Read the model definition and answer for the solid it produces. Units are mm, in the model's axes. A direction names the side the tool comes from. Give positions to 0.01 mm unless a question says otherwise; leave off trailing zeros. Order: outer loops, then holes, each group sorted by start corner. A loop starts at its lowest first (then second) coordinate and runs counter-clockwise, first axis right, second up. Notation, with made-up numbers: (62.5, 18.5) - (104.5, 18.5) arc R12 ccw to (104.5, 36.5) - close; hole circle Ø4 at (-12.5, 78). An arc over 180 degrees is marked (long way). Write each question's results on one line, items separated by ' | '. Start each with the question number.
Q1. A tool of negligible diameter and unlimited length cuts with its end or side. For faces 4 (the face through (0, 18.3, 0)), 5 (the face through (0.596, 5.315, -1.337)), 6 (the face through (-12, 1, 1.067)), from which of +Z, -Z, +X, -X, +Y, -Y can it reach the whole face along a straight path? Write none if from no direction.
Q2. Find the intervals of material crossed by line 1 along Y through (x, z) = (0, 1.45); line 2 along Y through (x, z) = (0, 0.25); line 3 along X through (y, z) = (1.75, 0.15), in increasing order. Write a range as from..to.
Q3. For a pull along Y with two mould halves and no side action, classify faces 1 (the face through (2.859, -2.797, -0.022)), 2 (the face through (-3, 6, -1.6)), 3 (the face through (-0.8, 15, 0)) as +Y half, -Y half, draft (parallel to the pull), parting line (faces both ways), or undercut.
Q4. Find section D-D on z = -0.1. Count the separate pieces of the cut face and the enclosed holes in it, and give its area (3 significant figures).
Q5. Find section A-A on x = -8. Give the vertices of the cut face in (y, z), and give its area (3 significant figures).
Q6. Flat-ended cylindrical pins translate along their axes: P1, Ø1.1, axis at y = -1.5, z = -0.5, coming from the -X side; P2, Ø0.7, axis at y = 17.5, z = -0.5, coming from the +X side; P3, Ø1.1, axis at y = -2, z = 0.5, coming from the +X side. Find the tip coordinate at first contact, or state that the pin passes through.
Q7. Find section C-C on x = -14.5. Give the vertices of the cut face in (y, z), and give its area (3 significant figures).
Autodesk Inventor part; units mm, degrees
ref_plane "YZ Plane" through (0, 0, 0) normal (1, 0, 0) x (0, 1, 0)
ref_plane "XZ Plane" through (0, 0, 0) normal (0, 1, 0) x (-1, 0, 0)
ref_plane "XY Plane" through (0, 0, 0) normal (0, 0, 1) x (1, 0, 0)
sketch "Sketch1" plane through (0, 0, 0) normal (0, 0, 1) x (1, 0, 0)
  line L0 (0, -9.7941) -> (0, 24.9657) construction
  line L1 (-24.9657, 0) -> (9.7941, 0) construction
  line L2 (-4, 4) -> (-4, 16)
  arc A0 (4, 16) -> (-4, 16) centre (0, 16) ccw
  line L3 (4, 16) -> (4, 0)
  arc A1 (0, -4) -> (4, 0) centre (0, 0) ccw
  line L4 (0, -4) -> (-16, -4)
  arc A2 (-16, 4) -> (-16, -4) centre (-16, 0) ccw
  line L5 (-16, 4) -> (-4, 4)
  dimension "d38" = 8
  dimension "d39" = 24
sketch "Sketch6" plane through (0, 0, 0) normal (0, 0, 1) x (1, 0, 0)
  circle A0 centre (-16, 0) radius 2.3
  circle A1 centre (0, 16) radius 2.3
  line L0 (-18.1564, 0.8) -> (-16.8, 0.8)
  line L1 (-16.8, 0.8) -> (-16.8, 2.1564)
  line L2 (-15.2, 2.1564) -> (-15.2, 0.8)
  line L3 (-15.2, 0.8) -> (-13.8436, 0.8)
  line L4 (-13.8436, -0.8) -> (-15.2, -0.8)
  line L5 (-15.2, -0.8) -> (-15.2, -2.1564)
  line L6 (-16.8, -2.1564) -> (-16.8, -0.8)
  line L7 (-16.8, -0.8) -> (-18.1564, -0.8)
  line L8 (-2.1564, 16.8) -> (-0.8, 16.8)
  line L9 (0.8, 16.8) -> (2.1564, 16.8)
  line L10 (0.8, 18.1564) -> (0.8, 16.8)
  line L11 (0.8, 15.2) -> (0.8, 13.8436)
  line L12 (-0.8, 18.1564) -> (-0.8, 16.8)
  line L13 (-0.8, 15.2) -> (-0.8, 13.8436)
  line L14 (2.1564, 15.2) -> (0.8, 15.2)
  line L15 (-0.8, 15.2) -> (-2.1564, 15.2)
  arc A2 (0, -4) -> (4, 0) centre (0, 0) ccw construction
  arc A3 (4, 16) -> (-4, 16) centre (0, 16) ccw construction
  arc A4 (-16, 4) -> (-16, -4) centre (-16, 0) ccw construction
  circle A5 centre (0, 0) radius 2.3
  line L16 (-2.1564, 0.8) -> (-0.8, 0.8)
  line L17 (-0.8, 0.8) -> (-0.8, 2.1564)
  line L18 (0.8, 2.1564) -> (0.8, 0.8)
  line L19 (0.8, 0.8) -> (2.1564, 0.8)
  line L20 (2.1564, -0.8) -> (0.8, -0.8)
  line L21 (0.8, -0.8) -> (0.8, -2.1564)
  line L22 (-0.8, -2.1564) -> (-0.8, -0.8)
  line L23 (-0.8, -0.8) -> (-2.1564, -0.8)
  circle A6 centre (0, 0) radius 2.75
  circle A7 centre (-16, 0) radius 2.75
  circle A8 centre (0, 16) radius 2.75
  dimension "d40" = 4.6
  dimension "d41" = 1.6
  dimension "d50" = 5.5
sketch "Sketch8" plane through (0, 0, 0) normal (0, 0, 1) x (1, 0, 0)
  arc A0 (0, -4) -> (4, 0) centre (0, 0) ccw construction
  line L0 (0, -8.9941) -> (0, 20.1657) construction
  line L1 (-20.1657, 0) -> (8.9941, 0) construction
  circle A1 centre (0, 8) radius 2.4
  circle A2 centre (-8, 0) radius 2.4
  circle A3 centre (0, 8) radius 2.75
  circle A4 centre (-8, 0) radius 2.75
  line L2 (0, -4) -> (-16, -4) construction
  line L3 (4, 16) -> (4, 0) construction
  point P0 (4, 8)
  point P1 (-8, -4)
  dimension "d42" = 4.8
  dimension "d43" = 5.5
extrude "Extrusion1" add sketch "Sketch1" along normal mid plane 3.2
extrude "Extrusion9" cut sketch "Sketch6" along normal through all both and the other way through all contours A0 L4 L5 L6 L7 L0 L1 L2 L3 | A1 L14 L11 L13 L15 L8 L12 L10 L9 | A5 L20 L21 L22 L23 L16 L17 L18 L19
extrude "Extrusion10" cut sketch "Sketch8" along normal through all both and the other way through all contours A1 | A2
sketch "Sketch3" plane through (0, 0, 1.6) normal (0, 0, 1) x (1, 0, 0)
  circle A0 centre (-8, 0) radius 2.75
  circle A1 centre (0, 8) radius 2.75
extrude "Extrusion4" cut sketch "Sketch3" against normal blind 0.5333
sketch "Sketch9" plane through (0, 0, -1.6) normal (0, 0, -1) x (-1, 0, 0)
  circle A0 centre (8, 0) radius 2.75
  circle A1 centre (0, 8) radius 2.75
extrude "Extrusion11" cut sketch "Sketch9" against normal blind 0.5333
sketch "Sketch4" plane through (0, 0, 1.6) normal (0, 0, 1) x (1, 0, 0)
  circle A0 centre (-16, 0) radius 2.3 construction
  circle A1 centre (0, 16) radius 2.3 construction
  arc A2 (-5.9892, -3.3333) -> (-5.9892, 3.3333) centre (-8, 0) ccw
  line L0 (-5.9892, 3.3333) -> (-2.0108, 3.3333)
  line L1 (-5.9892, -3.3333) -> (-2.0108, -3.3333)
  arc A3 (-2.0108, 3.3333) -> (-2.0108, -3.3333) centre (0, 0) ccw
  circle A4 centre (0, 0) radius 2.75 construction
  circle A5 centre (0, 16) radius 2.75 construction
  circle A6 centre (-16, 0) radius 2.75 construction
  line L2 (0, -9.5229) -> (0, 24.9205) construction
  line L3 (-25.4536, 0) -> (12.7217, 0) construction
  circle A7 centre (-8, 0) radius 2.75 construction
  circle A8 centre (0, 8) radius 2.75 construction
  arc A9 (-10.0108, 3.3333) -> (-10.0108, -3.3333) centre (-8, 0) ccw
  arc A10 (-13.9892, -3.3333) -> (-13.9892, 3.3333) centre (-16, 0) ccw
  line L4 (-10.0108, -3.3333) -> (-13.9892, -3.3333)
  line L5 (-10.0108, 3.3333) -> (-13.9892, 3.3333)
  arc A11 (3.3333, 2.0108) -> (-3.3333, 2.0108) centre (0, 0) ccw
  arc A12 (-3.3333, 5.9892) -> (3.3333, 5.9892) centre (0, 8) ccw
  line L6 (3.3333, 2.0108) -> (3.3333, 5.9892)
  line L7 (-3.3333, 2.0108) -> (-3.3333, 5.9892)
  line L8 (3.3333, 10.0108) -> (3.3333, 13.9892)
  line L9 (-3.3333, 10.0108) -> (-3.3333, 13.9892)
  arc A13 (-3.3333, 13.9892) -> (3.3333, 13.9892) centre (0, 16) ccw
  arc A14 (3.3333, 10.0108) -> (-3.3333, 10.0108) centre (0, 8) ccw
  dimension "d33" = 6.6667
  dimension "d51" = 1.1429
  dimension "d52" = 6.6667
extrude "Extrusion5" cut sketch "Sketch4" against normal blind 0.5333
sketch "Sketch10" plane through (0, 0, -1.6) normal (0, 0, -1) x (-1, 0, 0)
  arc A0 (-3.3333, 13.9892) -> (3.3333, 13.9892) centre (0, 16) ccw
  line L0 (3.3333, 13.9892) -> (3.3333, 10.0108)
  arc A1 (3.3333, 10.0108) -> (-3.3333, 10.0108) centre (0, 8) ccw
  line L1 (-3.3333, 10.0108) -> (-3.3333, 13.9892)
  arc A2 (2.0108, -3.3333) -> (-3.3333, 2.0108) centre (0, 0) ccw
  line L2 (-3.3333, 2.0108) -> (-3.3333, 5.9892)
  arc A3 (-3.3333, 5.9892) -> (3.3333, 5.9892) centre (0, 8) ccw
  line L3 (3.3333, 5.9892) -> (3.3333, 3.3333)
  line L4 (3.3333, 3.3333) -> (5.9892, 3.3333)
  arc A4 (5.9892, 3.3333) -> (5.9892, -3.3333) centre (8, 0) ccw
  line L5 (5.9892, -3.3333) -> (2.0108, -3.3333)
  line L6 (10.0108, 3.3333) -> (13.9892, 3.3333)
  arc A5 (13.9892, 3.3333) -> (13.9892, -3.3333) centre (16, 0) ccw
  line L7 (13.9892, -3.3333) -> (10.0108, -3.3333)
  arc A6 (10.0108, -3.3333) -> (10.0108, 3.3333) centre (8, 0) ccw
extrude "Extrusion12" cut sketch "Sketch10" against normal blind 0.5333
equation "\"d38\" = width_standard"
equation "\"d2\" = 0.333333 * height_standard"
equation "\"d15\" = 0.0555556 * height_standard"
equation "\"d48\" = 0.0555556 * height_standard"
equation "\"d33\" = 0.833333 * width_standard"
equation "\"d52\" = 0.833333 * width_standard"
equation "\"d20\" = 0.0555556 * height_standard"
equation "\"d53\" = 0.0555556 * height_standard"
equation "\"width_standard\" = 8"
equation "\"height_standard\" = 9.6"
properties part number "LEGO Brick 32017" material "Steel"
Working result:
1) face 4: +Z, -Z | face 5: -Z | face 6: +Z
2) line 1: -4..-2.3, 2.3..3.89, 4.11..5.25, 10.75..11.89, 12.11..13.7, 18.3..20 | line 2: -4..-2.3, 2.3..5.6, 10.4..13.7, 18.3..20 | line 3: -19.6..-16.8, -15.2..-9.64, -6.36..-0.8, 0.8..4
3) face 1: -Y half | face 2: draft | face 3: undercut
4) separate pieces: 1 | enclosed holes: 5 | area: 231 mm²
5) outline: (-4, -1.6) - (-2.75, -1.6) - (-2.75, -1.07) - (-2.4, -1.07) - (-2.4, 1.07) - (-2.75, 1.07) - (-2.75, 1.6) - (-4, 1.6) - close; (2.4, -1.07) - (2.75, -1.07) - (2.75, -1.6) - (4, -1.6) - (4, 1.6) - (2.75, 1.6) - (2.75, 1.07) - (2.4, 1.07) - close | area: 9.49 mm²
6) P1: x = -19.89 | P2: x = 3.83 | P3: x = 3.73
7) outline: (-4, -1.6) - (-0.8, -1.6) - (-0.8, 1.6) - (-4, 1.6) - close; (0.8, -1.6) - (4, -1.6) - (4, 1.6) - (0.8, 1.6) - close | area: 20.5 mm²
